```python
from build123d import *

# Parameters (mm, degrees)
SKETCH_1_W          = 45.7
SKETCH_1_H          = 25.4
EXTRUDE_1_DEPTH     = 21.5
EXTRUDE_1_TAPER     = 2
FILLET_1_R          = 1
SKETCH_2_R          = 0.6
EXTRUDE_2_DEPTH     = 3.5
CUT_EXTRUDE_1_DEPTH = 0.1


with BuildPart() as part:
    # Эскиз1 → Бобышка-Вытянуть1 (new body)
    with BuildSketch(Plane(origin=(0, 0, 0), x_dir=(1, 0, 0), z_dir=(0, 1, 0))):
        Rectangle(SKETCH_1_W, SKETCH_1_H)
    extrude(amount=EXTRUDE_1_DEPTH, taper=EXTRUDE_1_TAPER)

    # Скругление1
    fillet_1_edges = [part.edges().sort_by_distance(p)[0] for p in [
        (-22.099203456, 21.5, 0),
        (0, 21.5, 11.949203456),
        (22.099203456, 21.5, 0),
        (22.474601728, 10.75, 12.324601728),
        (-22.474601728, 10.75, 12.324601728),
        (-22.474601728, 10.75, -12.324601728),
        (22.474601728, 10.75, -12.324601728),
        (0, 21.5, -11.949203456),
    ]]
    fillet(fillet_1_edges, radius=FILLET_1_R)

    # Эскиз2 → Бобышка-Вытянуть2 (add)
    with BuildSketch(Plane.XZ):
        with Locations(Location((-19.25, 9.25, 0), (0, 0, 90))):
            Circle(SKETCH_2_R)
        with Locations(Location((19.25, 9.25, 0), (0, 0, 90))):
            Circle(SKETCH_2_R)
        with Locations(Location((19.25, 1.25, 0), (0, 0, 90))):
            Circle(SKETCH_2_R)
        with Locations(Location((-19.25, -1.5, 0), (0, 0, 90))):
            Circle(SKETCH_2_R)
    extrude(amount=EXTRUDE_2_DEPTH)

    # Эскиз3 → Вырез-Вытянуть1 (cut)
    with BuildSketch(Plane(origin=(0, 21.5, 0), x_dir=(1, 0, 0), z_dir=(0, 1, 0))):
        Polygon((19.640008188, -9.100397798), (19.055592603, -8.995892928), (19.055592603, -7.470933512), (19.640008188, -7.575438382), align=None)
        Polygon((20.289358837, -1.113384811), (18.925722473, -1.113384811), (18.925722473, -2.217280915), (18.341306889, -2.217280915), (18.341306889, -1.113384811), (16.977670525, -1.113384811), (16.977670525, -0.593904292), (18.341306889, -0.593904292), (18.341306889, 0.509991812), (18.925722473, 0.509991812), (18.925722473, -0.593904292), (20.289358837, -0.593904292), align=None)
        Polygon((-21.133514681, -6.373125071), (-16.133514681, -7.217280915), (-16.133514681, -7.742849097), (-20.549099097, -6.99711046), (-20.549099097, -9.165332863), (-21.133514681, -9.100397798), align=None)
        with BuildLine():
            Line((-21.133514681, 2.58791389), (-16.133514681, 1.733611942))
            Line((-16.133514681, 1.733611942), (-16.133514681, 1.185722332))
            Line((-16.133514681, 1.185722332), (-18.017646175, 0.50491876))
            add(Edge.make_bspline(
                [(-18.017646175, 0.50491876), (-18.084951638, 0.479901412), (-18.216446711, 0.431024873), (-18.409455405, 0.359102014), (-18.595117789, 0.294326278), (-18.771368832, 0.230303102), (-18.94005961, 0.173527591), (-19.099405054, 0.11756543), (-19.251272194, 0.068533592), (-19.349820298, 0.037152336), (-19.397516304, 0.021964215)],
                knots=[0, 0, 0, 0, 1.17864921, 2.302733803, 3.380832114, 4.40627524, 5.380631262, 6.302323787, 7.178346691, 8, 8, 8, 8], degree=3))
            add(Edge.make_bspline(
                [(-19.397516304, 0.021964215), (-19.466070769, 0.000654731), (-19.611110517, -0.044429456), (-19.843139107, -0.108631255), (-20.100830498, -0.176769053), (-20.281849123, -0.221474359), (-20.37661533, -0.244878317)],
                knots=[0, 0, 0, 0, 0.848709835, 1.795603867, 2.845962616, 4, 4, 4, 4], degree=3))
            add(Edge.make_bspline(
                [(-20.37661533, -0.244878317), (-20.158646903, -0.272468182), (-19.72000482, -0.327990331), (-19.28337221, -0.397574555), (-19.063709486, -0.43258124)],
                knots=[0, 0, 0, 0, 0.99383272, 2, 2, 2, 2], degree=3))
            Line((-19.063709486, -0.43258124), (-16.133514681, -0.940901045))
            Line((-16.133514681, -0.940901045), (-16.133514681, -1.468498447))
            Line((-16.133514681, -1.468498447), (-21.133514681, -0.622313382))
            Line((-21.133514681, -0.622313382), (-21.133514681, -0.074423772))
            Line((-21.133514681, -0.074423772), (-18.259123447, 0.965551877))
            add(Edge.make_bspline(
                [(-18.259123447, 0.965551877), (-18.13342725, 1.006165207), (-17.890654825, 1.084606694), (-17.5379298, 1.192033494), (-17.210066563, 1.286371648), (-16.998768155, 1.340422442), (-16.897516304, 1.366322981)],
                knots=[0, 0, 0, 0, 1.11654548, 2.156520707, 3.116625202, 4, 4, 4, 4], degree=3))
            add(Edge.make_bspline(
                [(-16.897516304, 1.366322981), (-16.98313031, 1.373970961), (-17.163429992, 1.390077303), (-17.446573636, 1.425294437), (-17.75612092, 1.470909488), (-17.970717493, 1.508204888), (-18.08258124, 1.527646033)],
                knots=[0, 0, 0, 0, 0.862057772, 1.815459291, 2.861254385, 4, 4, 4, 4], degree=3))
            Line((-18.08258124, 1.527646033), (-21.133514681, 2.062345708))
            Line((-21.133514681, 2.062345708), (-21.133514681, 2.58791389))
        make_face()
    extrude(amount=-CUT_EXTRUDE_1_DEPTH, mode=Mode.SUBTRACT)


solid = part.part
```
Work out the finished part from the listing and answer in its coordinate system (mm). A direction names the side the tool comes from. Round coordinates to 2 decimals unless told otherwise and drop trailing zeros.
(1) Each of these flat-tipped pins is pushed along its axis until it touches: P1, Ø5, axis at y = 7, z = -6.5, coming from the +X side; P2, Ø2, axis at x = 16.5, y = 18.5, coming from the +Z side; P3, Ø8, axis at x = 6.5, z = 4.5, coming from the -Y side. Where does it stop, or does it pass through?
Computed values:
P1: stops at x = 22.69
P2: stops at z = 12.09
P3: stops at y = 0
(2) Find the intervals of material crossed by L1, parallel to Y at x = 13.5, z = -3; L2, parallel to Z at x = 11, y = 0.25; L3, parallel to Y at x = 21.5, z = -4.5, in increasing order.
Computed values:
L1: y = 0 to 21.5
L2: z = -12.69 to 12.69
L3: y = 0 to 21.43
(3) For faces 1 (the cylindrical face through (-19.845, -1.726, 9.172)), 2 (the flat face through (-18.6, 21.4, -0.6)), 3 (the flat face through (19, -3.5, 1)), determine the directions among +Z, -Z, +X, -X, +Y, -Y from which every point of the face is accessible in a straight line to the end or side of a thin tool.
Computed values:
face 1: -Y
face 2: +Y
face 3: +Z, -Z, +X, -X, -Y
(4) The mould has two halves that part along X. Classify faces 4 (the cylindrical face through (18.655, -1.726, 9.172)), 5 (the cylindrical face through (-19.845, -1.726, -1.578)), 6 (the flat face through (-19.3, -3.5, -1.5)): pulls with the +X half, pulls with the -X half, needs draft (parallel to the pull), parting line crosses it, or undercut.
Computed values:
face 4: undercut
face 5: parting line crosses it
face 6: needs draft
